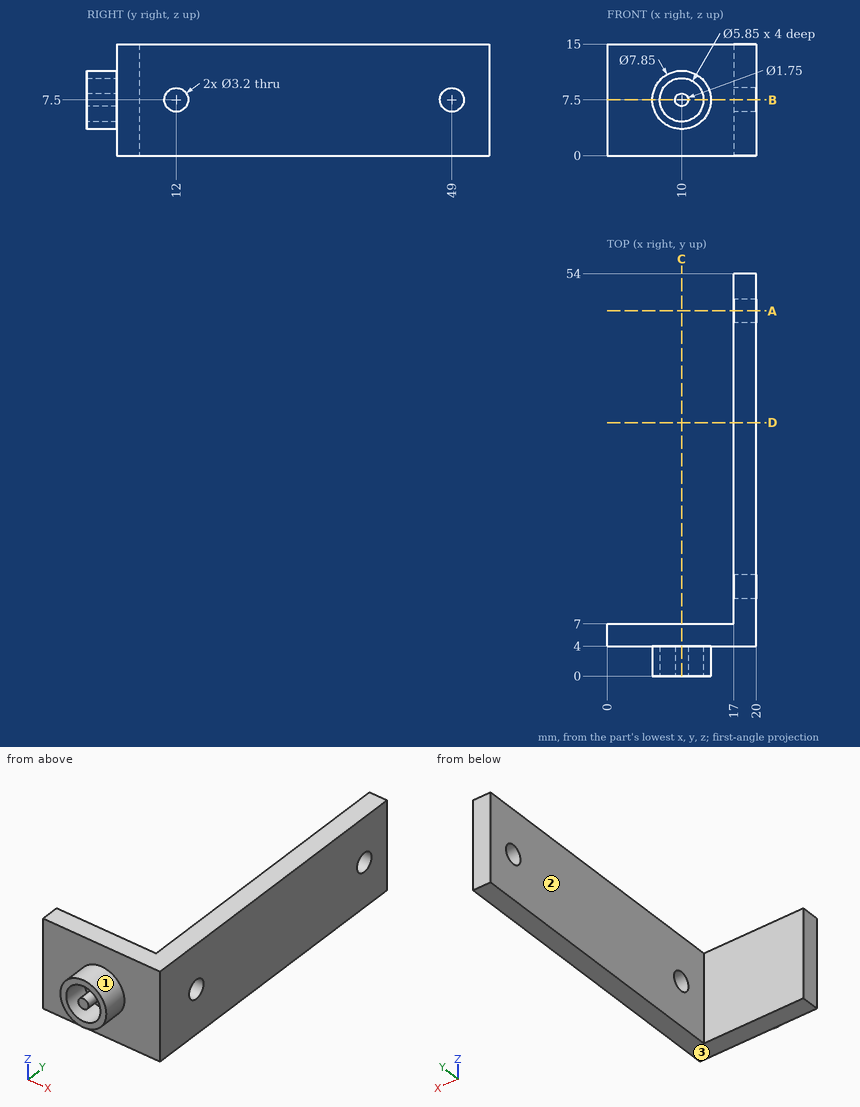
Study the drawing (mm; zero at the part's minimum x, y, z) and answer. A direction names the side the tool comes from. Give positions to 0.01 mm unless a question says otherwise; leave off trailing zeros. Loops run counter-clockwise (first coordinate to the right, second up) from the corner with the lowest first, then second, coordinate; pieces in that order, holes last. Notation, with made-up numbers: (36, 8) -> (57, 8) arc R9 ccw to (57, 22) -> close; hole circle Ø3 at (4, -8). An arc over 180 degrees is marked (long way). Use a Markdown table: item, result. Add a question column.
1) The part is cut by section A-A, the plane y = 49. Determine the outline of the cut face in (x, z), plus the area to 3 significant figures.
2) The part is cut by section C-C, the plane x = 10. Determine the outline of the cut face in (y, z) (3 decimals), plus the area to 3 significant figures.
3) The part is cut by section B-B, the plane z = 7.5. Determine the outline of the cut face in (x, y) (3 decimals).
4) The part is cut by section D-D, the plane y = 34. Determine the outline of the cut face in (x, z).
5) Each of these flat-tipped pins is pushed along its axis until it touches: P1, Ø1.5, axis at x = 13, z = 12.5, coming from the -Y side; P2, Ø2.5, axis at y = 12, z = 7.5, coming from the -X side; P3, Ø4.5, axis at x = 7, z = 8.5, coming from the +Y side; P4, Ø8, axis at y = 43.5, z = 9.5, coming from the -X side. Where does it stop, or does it pass through?
6) Consider line 1 along Y through (x, z) = (18.3, 7.5); line 2 along X through (y, z) = (1.5, 7.5) (3 decimals); line 3 along Y through (x, z) = (11, 7.5). Determine where each line is inside the solid, lowest interval first.
7) Which of the six approach directions +Z, -Z, +X, -X, +Y, -Y give full straight-line access (tool end or side, diameter ignored) to the marked faces 1, 2 and 3?
Reported:
| question | item | result |
|---|---|---|
| 1 | outline | (17, 0) -> (20, 0) -> (20, 5.9) -> (17, 5.9) -> close; (17, 9.1) -> (20, 9.1) -> (20, 15) -> (17, 15) -> close |
| 1 | area | 35.4 mm^2 |
| 2 | outline | (0, 3.575) -> (4, 3.575) -> (4, 0) -> (7, 0) -> (7, 15) -> (4, 15) -> (4, 11.425) -> (0, 11.425) -> (0, 10.425) -> (4, 10.425) -> (4, 8.375) -> (0, 8.375) -> (0, 6.625) -> (4, 6.625) -> (4, 4.575) -> (0, 4.575) -> close |
| 2 | area | 60.0 mm^2 |
| 3 | outline | (0, 4) -> (6.075, 4) -> (6.075, 0) -> (7.075, 0) -> (7.075, 4) -> (9.125, 4) -> (9.125, 0) -> (10.875, 0) -> (10.875, 4) -> (12.925, 4) -> (12.925, 0) -> (13.925, 0) -> (13.925, 4) -> (20, 4) -> (20, 10.4) -> (17, 10.4) -> (17, 7) -> (0, 7) -> close; (17, 13.6) -> (20, 13.6) -> (20, 47.4) -> (17, 47.4) -> close; (17, 50.6) -> (20, 50.6) -> (20, 54) -> (17, 54) -> close |
| 4 | outline | (17, 0) -> (20, 0) -> (20, 15) -> (17, 15) -> close |
| 5 | P1 | stops at y = 4 |
| 5 | P2 | passes through |
| 5 | P3 | stops at y = 7 |
| 5 | P4 | stops at x = 17 |
| 6 | line 1 | y = 4 to 10.4, 13.6 to 47.4, 50.6 to 54 |
| 6 | line 2 | x = 6.075 to 7.075, 9.125 to 10.875, 12.925 to 13.925 |
| 6 | line 3 | y = 4 to 7 |
| 7 | face 1 | -Y |
| 7 | face 2 | +Z, -Z, -X, +Y |
| 7 | face 3 | -Z, +X, -X, +Y, -Y |
